from build123d import *

# Parameters (mm, degrees)
SKETCH1_W           = 82.55
SKETCH1_H           = 44.45
BOSS_EXTRUDE1_DEPTH = 3.175
SKETCH2_R           = 2.54
CUT_EXTRUDE1_DEPTH  = 3.175
SKETCH4_W           = 54.61
SKETCH4_H           = 24.765
CUT_EXTRUDE2_DEPTH  = 3.175
SKETCH5_W           = 82.55
SKETCH5_H           = 3.175
BOSS_EXTRUDE2_DEPTH = 25.4
SKETCH7_W           = 3.204255847
SKETCH7_H           = 38.1
BOSS_EXTRUDE3_DEPTH = 25.4
SKETCH6_R           = 3.429
CUT_EXTRUDE3_DEPTH  = 99.014466407


with BuildPart() as part:
    # Sketch1 → Boss-Extrude1 (new body)
    with BuildSketch(Plane(origin=(0, 0, 0), x_dir=(1, 0, 0), z_dir=(0, 1, 0))):
        with Locations((41.275, 22.225)):
            Rectangle(SKETCH1_W, SKETCH1_H)
    extrude(amount=BOSS_EXTRUDE1_DEPTH)

    # Sketch2 → Cut-Extrude1 (cut)
    with BuildSketch(Plane(origin=(0, 3.175, 0), x_dir=(1, 0, 0), z_dir=(0, 1, 0))):
        with Locations(Location((9.525, 22.225, 0), (0, 0, 270))):
            Circle(SKETCH2_R)
        with Locations(Location((73.025, 22.225, 0), (0, 0, 90))):
            Circle(SKETCH2_R)
    extrude(amount=-CUT_EXTRUDE1_DEPTH, mode=Mode.SUBTRACT)

    # Sketch4 → Cut-Extrude2 (cut)
    with BuildSketch(Plane(origin=(0, 3.175, 0), x_dir=(1, 0, 0), z_dir=(0, 1, 0))):
        with Locations((41.275, 22.225)):
            Rectangle(SKETCH4_W, SKETCH4_H)
    extrude(amount=-CUT_EXTRUDE2_DEPTH, mode=Mode.SUBTRACT)

    # Sketch5 → Boss-Extrude2 (add)
    with BuildSketch(Plane(origin=(0, 3.175, 0), x_dir=(1, 0, 0), z_dir=(0, 1, 0))):
        with Locations((41.275, 42.8625)):
            Rectangle(SKETCH5_W, SKETCH5_H)
        with Locations((41.275, 1.5875)):
            Rectangle(SKETCH5_W, SKETCH5_H)
    extrude(amount=BOSS_EXTRUDE2_DEPTH)

    # Sketch7 → Boss-Extrude3 (add)
    with BuildSketch(Plane(origin=(0, 3.175, 0), x_dir=(1, 0, 0), z_dir=(0, 1, 0))):
        with Locations((1.602127924, 22.225)):
            Rectangle(SKETCH7_W, SKETCH7_H)
        with Locations((80.947872077, 22.225)):
            Rectangle(SKETCH7_W, SKETCH7_H)
    extrude(amount=BOSS_EXTRUDE3_DEPTH)

    # Sketch6 → Cut-Extrude3 (cut, through all)
    with BuildSketch(Plane(origin=(0, 0, -44.45), x_dir=(-1, 0, 0), z_dir=(0, 0, -1))):
        with Locations((-28.575, 19.05)):
            Circle(SKETCH6_R)
        with Locations((-53.975, 19.05)):
            Circle(SKETCH6_R)
    extrude(amount=-CUT_EXTRUDE3_DEPTH, mode=Mode.SUBTRACT)


solid = part.part
The listing builds one solid part. Answer for the finished solid, in the listing's coordinates (mm). A direction names the side the tool comes from. Coordinates: 2 decimals unless noted, no trailing zeros. Loops run counter-clockwise (first coordinate to the right, second up) from the corner with the lowest first, then second, coordinate; pieces in that order, holes last. Notation, with made-up numbers: (67, 10) -> (95, 10) arc R28 ccw to (95, 45) -> close; hole circle Ø2 at (20, -17.75). An arc over 180 degrees is marked (long way). Write item = value, one per line. Start each with the question number.
1) Straight lines are drawn through the part: line 1 (X direction, y = 15.5, z = -9.5); line 2 (Z direction, x = 7, y = 21.75) (3 decimals); line 3 (Z direction, x = 14, y = 2.75). For each, find the intervals that lie inside material, in ascending order. Write a range as from..to.
2) A tool of negligible diameter and unlimited length cuts with its end or side. For faces 1 (the face through (41, 2, -34.608)), 2 (the face through (41, 16, -3.175)), 3 (the face through (26.99, 16.01, -42.88)), from which of +Z, -Z, +X, -X, +Y, -Y can it reach the whole face along a straight path? Write none if from no direction.
3) A cutting plane is placed at A-A (y = 19.05). Give the vertices of the cut face in (x, z) (3 decimals).
4) Given pin 1 Ø5.5 at (x, y) = (53.975, 19.05) entering from -Z, flat-ended and moving along its own axis, determine where the tip first touches the part or whether it passes through.
5) A cutting plane is placed at D-D (y = 10). Give the vertices of the cut face in (x, z) (3 decimals).
6) The mould has two halves that part along Z. Classify faces 4 (the face through (41, 0, -8)), 5 (the face through (41, 2, -9.843)), 6 (the face through (41, 14, -44.45)), 7 (the face through (41, 14, 0)): released by +Z, released by -Z, zero draft, split by the parting line, or undercut.
7) A cutting plane is placed at C-C (x = 77). Give the vertices of the cut face in (y, z) (3 decimals), then the cut area to 3 significant figures.
Responses:
q1.line_1 = 0..3.2, 79.35..82.55
q1.line_2 = -44.45..-41.275, -3.175..0
q1.line_3 = -44.45..-34.61, -9.84..0
q2.face_1 = +Y, -Y
q2.face_2 = +Y
q2.face_3 = +Z, -Z
q3.outline = (0, -44.45) -> (25.146, -44.45) -> (25.146, -41.275) -> (3.204, -41.275) -> (3.204, -3.175) -> (25.146, -3.175) -> (25.146, 0) -> (0, 0) -> close; (32.004, -44.45) -> (50.546, -44.45) -> (50.546, -41.275) -> (32.004, -41.275) -> close; (32.004, -3.175) -> (50.546, -3.175) -> (50.546, 0) -> (32.004, 0) -> close; (57.404, -44.45) -> (82.55, -44.45) -> (82.55, 0) -> (57.404, 0) -> (57.404, -3.175) -> (79.346, -3.175) -> (79.346, -41.275) -> (57.404, -41.275) -> close
q4.pin_1 = through
q5.outline = (0, -44.45) -> (82.55, -44.45) -> (82.55, 0) -> (0, 0) -> close; hole (3.204, -41.275) -> (79.346, -41.275) -> (79.346, -3.175) -> (3.204, -3.175) -> close
q6.face_4 = zero draft
q6.face_5 = undercut
q6.face_6 = released by -Z
q6.face_7 = released by +Z
q7.outline = (0, -44.45) -> (28.575, -44.45) -> (28.575, -41.275) -> (3.175, -41.275) -> (3.175, -3.175) -> (28.575, -3.175) -> (28.575, 0) -> (0, 0) -> close
q7.area = 302 mm²
